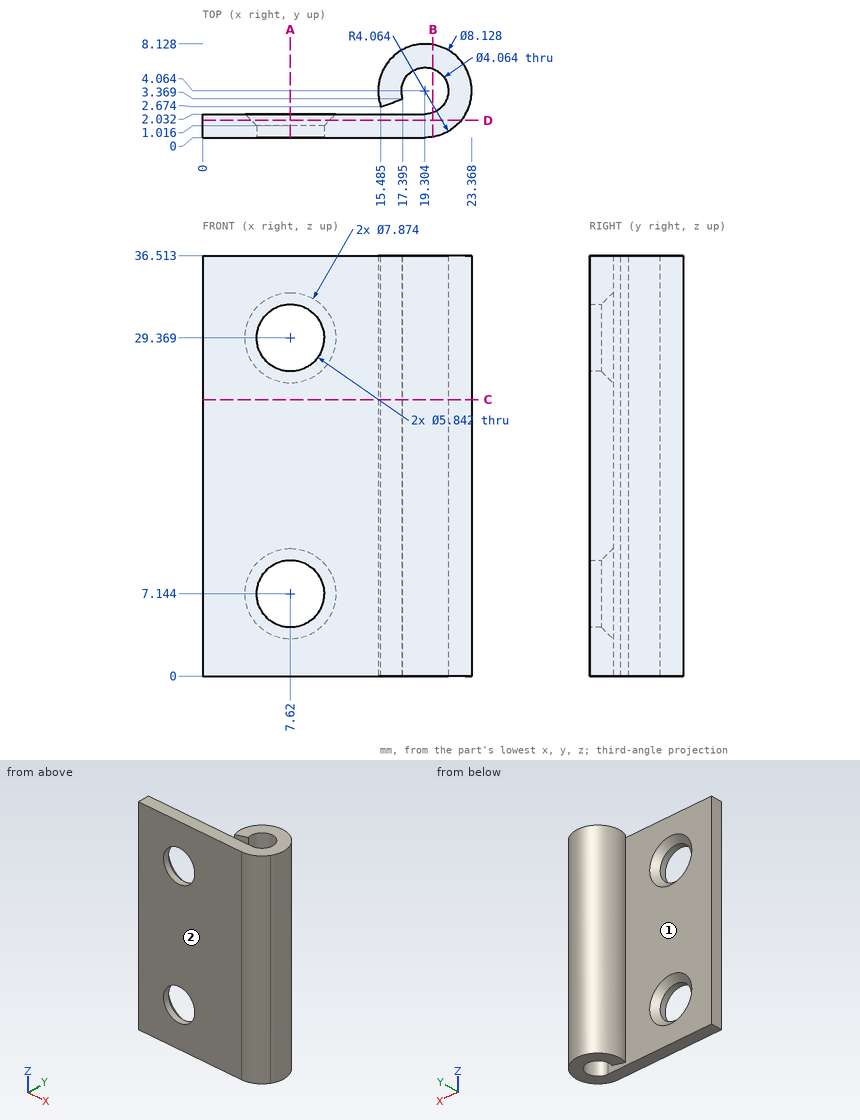
Design review of the part shown in the three views and the two pictorial views. Dimensions are in mm from the part's minimum x, y and z. A direction names the side the tool comes from. Coordinates: 2 decimals unless noted, no trailing zeros. Loops run counter-clockwise (first coordinate to the right, second up) from the corner with the lowest first, then second, coordinate; pieces in that order, holes last.
Q1. Tool access review of the marked faces 1 and 2: name each direction out of +Z, -Z, +X, -X, +Y, -Y from which nothing blocks a thin tool from reaching the whole face with its end or side.
Reported:
face 1: +Z, -Z, -X
face 2: +Z, -Z, +X, -X, -Y
Q2. We need section C-C on z = 24. State the section outline as (x, y) points (1 decimal).
Reported:
outline: (0, 0) - (19.3, 0) arc R4.1 ccw (long way) to (15.5, 2.7) - (17.4, 3.4) arc R2 cw (long way) to (19.3, 2) - (0, 2) - close
Q3. To check wall thickness, follow line 1 (Y direction, x = 2.75, z = 22); line 2 (X direction, y = 4, z = 23.5) (1 decimal); line 3 (X direction, y = 3.75, z = 15.5) (1 decimal). State the ranges of each line that lie inside material, in increasing order.
Reported:
line 1: y = 0 to 2.03
line 2: x = 15.2 to 17.3, 21.3 to 23.4
line 3: x = 15.3 to 17.3, 21.3 to 23.4
Q4. We need section A-A on x = 7.62. State the section outline as (y, z) points (1 decimal).
Reported:
outline: (0, 0) - (2, 0) - (2, 3.2) - (1, 4.2) - (0, 4.2) - close; (0, 10.1) - (1, 10.1) - (2, 11.1) - (2, 25.4) - (1, 26.4) - (0, 26.4) - close; (0, 32.3) - (1, 32.3) - (2, 33.3) - (2, 36.5) - (0, 36.5) - close
Q5. For pin 1 (4 mm diameter, centred on y = 6.5, z = 27.5, fed in from +X) (1 decimal); pin 2 (5.5 mm diameter, centred on x = 7.62, z = 7.14, fed in from -Y); pin 3 (1 mm diameter, centred on y = 6.5, z = 27, fed in from -X); pin 4 (9.5 mm diameter, centred on x = 7.62, z = 29.37, fed in from +Y), all flat-tipped, find the tip position at first contact; note any pin that passes through.
Reported:
pin 1: stops at x = 23.3
pin 2: passes through
pin 3: stops at x = 15.73
pin 4: stops at y = 2.03
Q6. We need section D-D on y = 1.5. State the section outline as (x, z) points (1 decimal), and give its area (3 significant figures).
Reported:
outline: (0, 0) - (22.5, 0) - (22.5, 36.5) - (0, 36.5) - close; hole circle Ø6.8 at (7.6, 7.1); hole circle Ø6.8 at (7.6, 29.4)
area: 747 mm2
Q7. We need section B-B on x = 20. State the section outline as (y, z) points (1 decimal), and give its area (3 significant figures).
Reported:
outline: (0.1, 0) - (2.2, 0) - (2.2, 36.5) - (0.1, 36.5) - close; (6, 0) - (8.1, 0) - (8.1, 36.5) - (6, 36.5) - close
area: 153 mm2
